```python
from build123d import *

# Parameters (mm, degrees)
SKETCH1_W           = 32
SKETCH1_H           = 34.5
SKETCH1_R           = 1.5
BOSS_EXTRUDE1_DEPTH = 2
SKETCH2_R           = 2
BOSS_EXTRUDE2_DEPTH = 5
FILLET1_R           = 1.2


with BuildPart() as part:
    # Sketch1 → Boss-Extrude1 (new body)
    with BuildSketch(Plane.XY):
        Rectangle(SKETCH1_W, SKETCH1_H)
        with Locations((-13.5, 14.75)):
            Circle(SKETCH1_R, mode=Mode.SUBTRACT)
        with Locations((13.5, 14.75)):
            Circle(SKETCH1_R, mode=Mode.SUBTRACT)
        with Locations((-13.5, -14.75)):
            Circle(SKETCH1_R, mode=Mode.SUBTRACT)
        with Locations((13.5, -14.75)):
            Circle(SKETCH1_R, mode=Mode.SUBTRACT)
    extrude(amount=BOSS_EXTRUDE1_DEPTH)

    # Sketch2 → Boss-Extrude2 (add)
    with BuildSketch(Plane.XY.offset(2)):
        with Locations((-10, 11.75)):
            Circle(SKETCH2_R)
        with Locations((-5.2, 11.75)):
            Circle(SKETCH2_R)
        with Locations((-0.4, 11.75)):
            Circle(SKETCH2_R)
        with Locations((4.4, 11.75)):
            Circle(SKETCH2_R)
    extrude(amount=BOSS_EXTRUDE2_DEPTH)

    # Fillet1
    fillet1_edges = [part.edges().sort_by_distance(p)[0] for p in [
        (-12, 11.75, 7),
        (-7.2, 11.75, 7),
        (-2.4, 11.75, 7),
        (2.4, 11.75, 7),
    ]]
    fillet(fillet1_edges, radius=FILLET1_R)


solid = part.part
```
The listing builds one solid part. Answer for the finished solid, in the listing's coordinates (mm). A direction names the side the tool comes from. Round coordinates to 2 decimals unless told otherwise and drop trailing zeros. Write each loop counter-clockwise with the first axis right and the second up, starting at its lowest first coordinate (ties: lowest second). Pieces come first, ordered by that corner, then holes. Notation, with made-up numbers: (34, 74) -> (87, 74) arc R20 cw to (87, 81) -> close; hole circle Ø5 at (70, 60.25). An arc over 180 degrees is marked (long way). Use CSV: the item, a comma, the result in double quotes. Start each with the question number.
(1) Section C-C on z = 0.5 is taken. Give the vertices of the cut face in (x, y).
(2) Section D-D on z = 2.5 is taken. Give the vertices of the cut face in (x, y), then the cut area to 3 significant figures.
(3) Which of the six approach directions +Z, -Z, +X, -X, +Y, -Y give full straight-line access (tool end or side, diameter ignored) to faces 1 (the face through (-5, 12, 7)), 2 (the face through (-5.46, 13.733, 3.873))?
(4) Section A-A on y = -14.75 is taken. Give the vertices of the cut face in (x, z), then the cut area to 3 significant figures.
(5) Each of these flat-tipped pins is pushed along its axis until it touches: pin 1 (2 mm diameter, centred on x = -3, y = -2.5, fed in from +Z); pin 2 (2.5 mm diameter, centred on x = -13.5, y = 14.75, fed in from -Z). Where does it stop, or does it pass through?
(6) The mould has two halves that part along X. Classify faces 3 (the face through (12, -14.7, 1)), 4 (the face through (0, 12, 7)), 5 (the face through (-16, 0, 1)): released by +X, released by -X, zero draft, split by the parting line, or undercut.
(7) Section B-B on x = -13.5 is taken. Give the vertices of the cut face in (y, z).
(8) Consider L1, parallel to Y at x = -13.5, z = 0.7; L2, parallel to X at y = 10, z = 4.75; L3, parallel to Z at x = 1.5, y = -11. Determine where each line is inside the solid, lowest interval first. Write a range as from..to.
A:
1,outline,"(-16, -17.25) -> (16, -17.25) -> (16, 17.25) -> (-16, 17.25) -> close; hole circle Ø3 at (-13.5, -14.75); hole circle Ø3 at (-13.5, 14.75); hole circle Ø3 at (13.5, -14.75); hole circle Ø3 at (13.5, 14.75)"
2,outline,"circle Ø4 at (-10, 11.75); circle Ø4 at (-5.2, 11.75); circle Ø4 at (-0.4, 11.75); circle Ø4 at (4.4, 11.75)"
2,area,"50.3 mm²"
3,face 1,"+Z, +X, -X, +Y, -Y"
3,face 2,"+Z"
4,outline,"(-16, 0) -> (-15, 0) -> (-15, 2) -> (-16, 2) -> close; (-12, 0) -> (12, 0) -> (12, 2) -> (-12, 2) -> close; (15, 0) -> (16, 0) -> (16, 2) -> (15, 2) -> close"
4,area,"52.0 mm²"
5,pin 1,"stops at z = 2"
5,pin 2,"passes through"
6,face 3,"undercut"
6,face 4,"zero draft"
6,face 5,"released by -X"
7,outline,"(-17.25, 0) -> (-16.25, 0) -> (-16.25, 2) -> (-17.25, 2) -> close; (-13.25, 0) -> (13.25, 0) -> (13.25, 2) -> (-13.25, 2) -> close; (16.25, 0) -> (17.25, 0) -> (17.25, 2) -> (16.25, 2) -> close"
8,L1,"y = -17.25..-16.25, -13.25..13.25, 16.25..17.25"
8,L2,"x = -10.97..-9.03, -6.17..-4.23, -1.37..0.57, 3.43..5.37"
8,L3,"z = 0..2"
